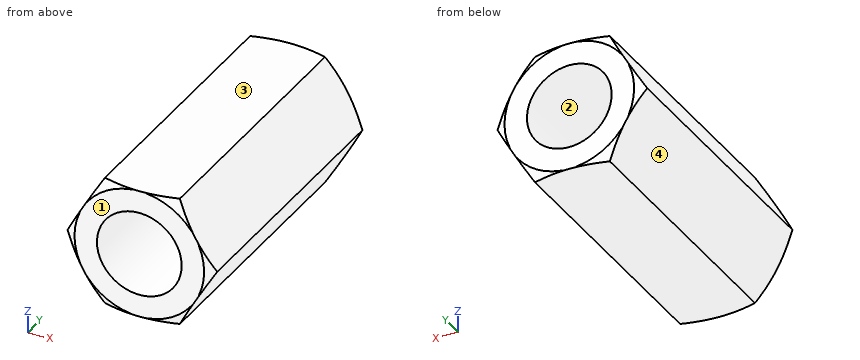
```python
from build123d import *

# Parameters (mm, degrees)
SKETCH_1_R          = 1.5
EXTRUDE_1_DEPTH     = 10
SKETCH_2_OUTSIDE_W  = 49.914
SKETCH_2_OUTSIDE_H  = 49.204
SKETCH_2_OUTSIDE_R  = 2.29496732
CUT_EXTRUDE_1_DEPTH = 11.596668108
CUT_EXTRUDE_1_DRAFT = -60
SKETCH_3_OUTSIDE_W  = 49.914
SKETCH_3_OUTSIDE_H  = 49.204
SKETCH_3_OUTSIDE_R  = 2.29496732
CUT_EXTRUDE_2_DEPTH = 11.596668108
CUT_EXTRUDE_2_DRAFT = -60


with BuildPart() as part:
    # Sketch 1 → Extrude 1 (new body)
    with BuildSketch(Plane(origin=(0, 0, 0), x_dir=(1, 0, 0), z_dir=(0, 1, 0))):
        Polygon((1.325, 2.29496732), (-1.325, 2.29496732), (-2.65, 0), (-1.325, -2.29496732), (1.325, -2.29496732), (2.65, 0), align=None)
        with Locations(Location((0, 0, 0), (0, 0, 270))):
            Circle(SKETCH_1_R, mode=Mode.SUBTRACT)
    extrude(amount=EXTRUDE_1_DEPTH)


with BuildPart() as cut_extrude_1_tool:
    # Sketch 2 outside → Cut-Extrude 1 (with draft: the straight prism first)
    with BuildSketch(Plane.XZ):
        Rectangle(SKETCH_2_OUTSIDE_W, SKETCH_2_OUTSIDE_H)
        Circle(SKETCH_2_OUTSIDE_R, mode=Mode.SUBTRACT)
    extrude(amount=-CUT_EXTRUDE_1_DEPTH)
    # Cut-Extrude 1: the draft: its side faces are tilted about the plane it starts from
    cut_extrude_1_sides = [cut_extrude_1_tool.faces().sort_by_distance(p)[0] for p in [
        (0, 5.798334054, -24.602),
        (24.957, 5.798334054, 0),
        (0, 5.798334054, 24.602),
        (-24.957, 5.798334054, 0),
        (-2.29496732, 5.798334054, 0),
    ]]
    draft(cut_extrude_1_sides, Plane.XZ, CUT_EXTRUDE_1_DRAFT)


with BuildPart() as part_1:
    add(part.part)

    # Cut-Extrude 1: cut by cut_extrude_1_tool
    add(cut_extrude_1_tool.part, mode=Mode.SUBTRACT)


with BuildPart() as cut_extrude_2_tool:
    # Sketch 3 outside → Cut-Extrude 2 (with draft: the straight prism first)
    with BuildSketch(Plane(origin=(0, 10, 0), x_dir=(1, 0, 0), z_dir=(0, 1, 0))):
        Rectangle(SKETCH_3_OUTSIDE_W, SKETCH_3_OUTSIDE_H)
        Circle(SKETCH_3_OUTSIDE_R, mode=Mode.SUBTRACT)
    extrude(amount=-CUT_EXTRUDE_2_DEPTH)
    # Cut-Extrude 2: the draft: its side faces are tilted about the plane it starts from
    cut_extrude_2_sides = [cut_extrude_2_tool.faces().sort_by_distance(p)[0] for p in [
        (0, 4.201665946, 24.602),
        (24.957, 4.201665946, 0),
        (0, 4.201665946, -24.602),
        (-24.957, 4.201665946, 0),
        (-2.29496732, 4.201665946, 0),
    ]]
    draft(cut_extrude_2_sides, Plane(origin=(0, 10, 0), x_dir=(1, 0, 0), z_dir=(0, 1, 0)), CUT_EXTRUDE_2_DRAFT)


with BuildPart() as part_2:
    add(part_1.part)

    # Cut-Extrude 2: cut by cut_extrude_2_tool
    add(cut_extrude_2_tool.part, mode=Mode.SUBTRACT)


solid = part_2.part
```
The model under review builds one solid part; all positions refer to its coordinate system, in mm. Face numbers are marked on the shaded views. Give positions to 0.01 mm unless a question says otherwise; leave off trailing zeros. Write each loop counter-clockwise with the first axis right and the second up, starting at its lowest first coordinate (ties: lowest second). Pieces come first, ordered by that corner, then holes. Notation, with made-up numbers: (51.5, 79.25) - (96.5, 79.25) arc R29 ccw to (96.5, 116.25) - close; hole circle Ø11 at (-24, 60). An arc over 180 degrees is marked (long way). Answer in a Markdown table with one row per item. Add a question column.
1. We need section A-A on y = 1.5. Write out the cut boundary in (x, z) (3 decimals).
2. Draft analysis for pull direction Z (two halves, no side actions). For the marked faces 1, 2, 3 and 4, state which applies: +Z half, -Z half, draft (parallel to the pull), parting line (faces both ways), or undercut.
3. Wall thickness on line 1 along X through (y, z) = (2.75, -1.35); line 2 along Z through (x, y) = (0.65, 7.25); line 3 along X through (y, z) = (1.25, 0.4): over which ranges is each line inside the solid? List them lowest first. Write a range as [from, to].
Ans:
| question | item | result |
|---|---|---|
| 1 | outline | (-2.65, 0) - (-1.325, -2.295) - (1.325, -2.295) - (2.65, 0) - (1.325, 2.295) - (-1.325, 2.295) - close; hole circle Ø3 at (0, 0) |
| 2 | face 1 | draft |
| 2 | face 2 | undercut |
| 2 | face 3 | +Z half |
| 2 | face 4 | -Z half |
| 3 | line 1 | x = [-1.87, -0.65], [0.65, 1.87] |
| 3 | line 2 | z = [-2.29, -1.35], [1.35, 2.29] |
| 3 | line 3 | x = [-2.42, -1.45], [1.45, 2.42] |
